The listing builds one solid part. Answer for the finished solid, in the listing's coordinates (mm). Face numbers are marked on the shaded views. A direction names the side the tool comes from. Coordinates: 2 decimals unless noted, no trailing zeros. Loops run counter-clockwise (first coordinate to the right, second up) from the corner with the lowest first, then second, coordinate; pieces in that order, holes last. Notation, with made-up numbers: M 16.25,40.5 L 69.25,40.5 A18 ccw 69.25,65.5 Z; hole C -19.5,67 d8. An arc over 180 degrees is marked long. Return JSON: item names as keys, results as strings. Group by question number.
1. The mould has two halves that part along X. Classify the marked faces 3, 4 and 5: pulls with the +X half, pulls with the -X half, needs draft (parallel to the pull), parting line crosses it, or undercut.
2. Section D-D (z = -3.5) is taken. Write down the section's boundary in (x, y).
3. Section C-C (x = -50) is taken. Write down the section's boundary in (y, z).
4. Straight lines are drawn through the part: L1, parallel to Y at x = 40.5, z = 35.5; L2, parallel to X at y = 12, z = -2.5; L3, parallel to X at y = 12, z = 7.5. For each, find the intervals that lie inside material, in ascending order. Write a range as from..to.
5. Section B-B (z = 15) is taken. Write down the section's boundary in (x, y), then the cut area to 3 significant figures.
6. Given P1, Ø3, axis at y = 25.5, z = -4, coming from the -X side; P2, Ø6, axis at x = -42.5, y = 19.5, coming from the +Z side; P3, Ø5, axis at x = -10, y = 21, coming from the -Z side, each flat-ended and moving along its own axis, determine where each tip first touches the part or whether it passes through.
7. Section A-A (y = 21) is taken. Write down the section's boundary in (x, z).
8. Which of the six approach directions +Z, -Z, +X, -X, +Y, -Y give full straight-line access (tool end or side, diameter ignored) to the marked faces 1 and 2?
```python
from build123d import *

# Parameters (mm, degrees)
BOSS_EXTRUDE1_DEPTH = 5
BOSS_EXTRUDE2_DEPTH = 20.3
BOSS_EXTRUDE3_DEPTH = 5
BOSS_EXTRUDE4_DEPTH = 20.3
BOSS_EXTRUDE5_DEPTH = 20.3


with BuildPart() as part:
    # Sketch2 → Boss-Extrude1 (new body)
    with BuildSketch(Plane(origin=(0, 0, 0), x_dir=(1, 0, 0), z_dir=(0, 1, 0))):
        Polygon((-56.59752525, -32.199536264), (0, 41.559794682), (0, -47.601200417), (-36.525685741, -47.601200417), align=None)
    boss_extrude1 = extrude(amount=BOSS_EXTRUDE1_DEPTH)

    # Sketch4 → Boss-Extrude2 (add)
    with BuildSketch(Plane(origin=(0, 5, 0), x_dir=(1, 0, 0), z_dir=(0, 1, 0))):
        Polygon((-56.59752525, -32.199536264), (-52.630758548, -35.243343409), (0, 33.346396524), (0, 41.559794682), align=None)
    boss_extrude2 = extrude(amount=BOSS_EXTRUDE2_DEPTH)

    # Sketch5 → Boss-Extrude3 (add)
    with BuildSketch(Plane(origin=(0, 25.3, 0), x_dir=(1, 0, 0), z_dir=(0, 1, 0))):
        Polygon((-56.59752525, -32.199536264), (-36.525685741, -47.601200417), (0, -47.601200417), (0, 41.559794682), align=None)
    boss_extrude3 = extrude(amount=BOSS_EXTRUDE3_DEPTH)

    # Sketch6 → Boss-Extrude4 (add)
    with BuildSketch(Plane(origin=(0, 5, 0), x_dir=(1, 0, 0), z_dir=(0, 1, 0))):
        Polygon((-17.031549002, 11.150449726), (0, -1.91831747), (0, 33.346396524), align=None)
    boss_extrude4 = extrude(amount=BOSS_EXTRUDE4_DEPTH)

    # Sketch7 → Boss-Extrude5 (add)
    with BuildSketch(Plane(origin=(0, 5, 0), x_dir=(1, 0, 0), z_dir=(0, 1, 0))):
        Polygon((-36.525685741, -47.601200417), (-0.926476194, -1.207407283), (0, -1.91831747), (0, -47.601200417), align=None)
    boss_extrude5 = extrude(amount=BOSS_EXTRUDE5_DEPTH)

    # Mirror2: Boss-Extrude1, Boss-Extrude2, Boss-Extrude3, Boss-Extrude4, Boss-Extrude5 across plane
    add(boss_extrude1.mirror(Plane(origin=(0, 5, -41.559794682), x_dir=(0, 0, 1), z_dir=(-1, 0, 0))))
    add(boss_extrude2.mirror(Plane(origin=(0, 5, -41.559794682), x_dir=(0, 0, 1), z_dir=(-1, 0, 0))))
    add(boss_extrude3.mirror(Plane(origin=(0, 5, -41.559794682), x_dir=(0, 0, 1), z_dir=(-1, 0, 0))))
    add(boss_extrude4.mirror(Plane(origin=(0, 5, -41.559794682), x_dir=(0, 0, 1), z_dir=(-1, 0, 0))))
    add(boss_extrude5.mirror(Plane(origin=(0, 5, -41.559794682), x_dir=(0, 0, 1), z_dir=(-1, 0, 0))))


solid = part.part
```
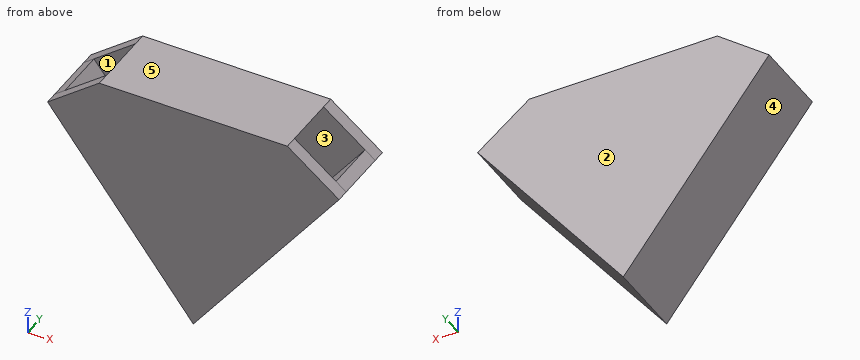
Worked out:
{
 "1": {"face 3": "undercut", "face 4": "pulls with the -X half", "face 5": "needs draft"},
 "2": {"outline": "M -29.2,0 L 29.2,0 L 29.2,30.3 L -29.2,30.3 Z; hole M -22.9,5 L -7.06,5 L -7.06,25.3 L -22.9,25.3 Z; hole M 7.06,5 L 22.9,5 L 22.9,25.3 L 7.06,25.3 Z"},
 "3": {"outline": "M 0,23.6 L 30.3,23.6 L 30.3,37.26 L 25.3,37.26 L 25.3,31.81 L 5,31.81 L 5,37.26 L 0,37.26 Z"},
 "4": {"L1": "0..5, 25.3..30.3", "L2": "-29.97..-23.67, -5.76..5.76, 23.67..29.97", "L3": "-37.64..-31.34, -5.75..5.75, 31.34..37.64"},
 "5": {"outline": "M -43.4,0 L 43.4,0 L 43.4,30.3 L -43.4,30.3 Z; hole M -37.1,5 L -11.51,5 L -11.51,25.3 L -37.1,25.3 Z; hole M 11.51,5 L 37.1,5 L 37.1,25.3 L 11.51,25.3 Z", "area": "1,590 mm^2"},
 "6": {"P1": "x = -29.97", "P2": "z = 25.95", "P3": "z = -31.79"},
 "7": {"outline": "M -56.6,32.2 L 0,-41.56 L 56.6,32.2 L 52.63,35.24 L 17.03,-11.15 L 0.93,1.21 L 36.53,47.6 L -36.53,47.6 L -0.93,1.21 L -17.03,-11.15 L -52.63,35.24 Z"},
 "8": {"face 1": "none", "face 2": "+Z, -Z, +X, -X, +Y"}
}
